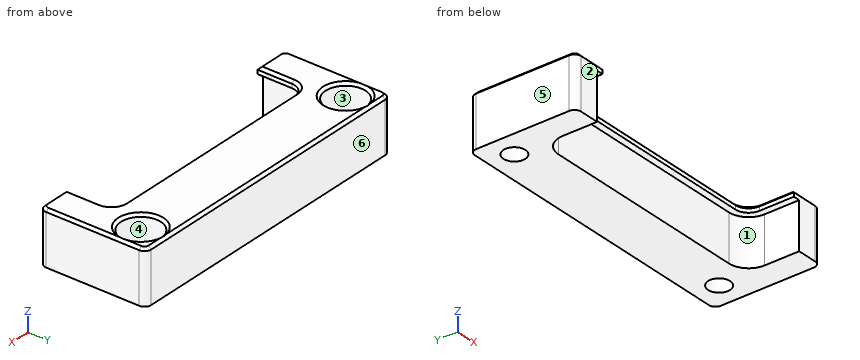
from build123d import *

# Parameters (mm, degrees)
BOSS_EXTRUDE1_DEPTH = 8
CUT_EXTRUDE1_REACH  = 51.356
SKETCH2_R           = 1.65
SKETCH3_R           = 3
CUT_EXTRUDE2_DEPTH  = 4.5
CUT_EXTRUDE3_DEPTH  = 7
FILLET1_R           = 1
CHAMFER2_SIZE       = 0.4


with BuildPart() as part:
    # Sketch1 → Boss-Extrude1 (new body)
    with BuildSketch(Plane.XY):
        with BuildLine():
            Line((0, 0), (0, 16))
            Line((0, 16), (46, 16))
            Line((46, 16), (46, 0))
            Line((46, 0), (41, 0))
            Line((41, 0), (41, 5.2))
            ThreePointArc((41, 5.2), (40.414213562, 6.614213562), (39, 7.2))
            Line((39, 7.2), (7, 7.2))
            ThreePointArc((7, 7.2), (5.585786438, 6.614213562), (5, 5.2))
            Line((5, 5.2), (5, 0))
            Line((5, 0), (0, 0))
        make_face()
    extrude(amount=BOSS_EXTRUDE1_DEPTH)

    # Sketch2 → Cut-Extrude1 (cut, up to next)
    with BuildSketch(Plane.XY.offset(8), mode=Mode.PRIVATE) as cut_extrude1_sk1:
        with Locations((3.75, 12.25)):
            Circle(SKETCH2_R)
    cut_extrude1_tool1 = extrude(cut_extrude1_sk1.sketch, amount=-CUT_EXTRUDE1_REACH, mode=Mode.PRIVATE) & part.part
    # Sketch2 → Cut-Extrude1 (cut, up to next)
    with BuildSketch(Plane.XY.offset(8), mode=Mode.PRIVATE) as cut_extrude1_sk2:
        with Locations((42.25, 12.25)):
            Circle(SKETCH2_R)
    cut_extrude1_tool2 = extrude(cut_extrude1_sk2.sketch, amount=-CUT_EXTRUDE1_REACH, mode=Mode.PRIVATE) & part.part
    add(cut_extrude1_tool1.solids().sort_by_distance((3.75, 12.25, 8))[0], mode=Mode.SUBTRACT)
    add(cut_extrude1_tool2.solids().sort_by_distance((42.25, 12.25, 8))[0], mode=Mode.SUBTRACT)

    # Sketch3 → Cut-Extrude2 (cut)
    with BuildSketch(Plane.XY.offset(8)):
        with Locations((3.75, 12.25)):
            Circle(SKETCH3_R)
        with Locations((42.25, 12.25)):
            Circle(SKETCH3_R)
    extrude(amount=-CUT_EXTRUDE2_DEPTH, mode=Mode.SUBTRACT)

    # Sketch4 → Cut-Extrude3 (cut)
    with BuildSketch(Plane(origin=(0, 0, 0), x_dir=(-1, 0, 0), z_dir=(0, 0, -1))):
        with BuildLine():
            Line((-4, 0), (-5, 0))
            Line((-5, 0), (-5, 5.2))
            ThreePointArc((-5, 5.2), (-5.585786438, 6.614213562), (-7, 7.2))
            Line((-7, 7.2), (-39, 7.2))
            ThreePointArc((-39, 7.2), (-40.414213592, 6.614213592), (-41, 5.2))
            Line((-41, 5.2), (-41, 0))
            Line((-41, 0), (-42, 0))
            Line((-42, 0), (-42, 5.200000101))
            ThreePointArc((-42, 5.200000101), (-41.121320373, 7.321320373), (-39.000000101, 8.2))
            Line((-39.000000101, 8.2), (-7, 8.2))
            ThreePointArc((-7, 8.2), (-4.878679656, 7.321320344), (-4, 5.2))
            Line((-4, 5.2), (-4, 0))
        make_face()
    extrude(amount=-CUT_EXTRUDE3_DEPTH, mode=Mode.SUBTRACT)

    # Fillet1
    fillet1_edges = [part.edges().sort_by_distance(p)[0] for p in [
        (0, 0, 4),
        (0, 16, 4),
        (46, 16, 4),
        (46, 0, 4),
    ]]
    fillet(fillet1_edges, radius=FILLET1_R)

    # Chamfer2
    # the kernel refuses this chamfer: 0.4 mm, written as the material it takes off along each edge
    with BuildSketch(Plane(origin=(6.028673195, 0, 8), x_dir=(0, 0.9996219169112966, 0.027495876610587326), z_dir=(-1, 0, 0)), Plane(origin=(45, 0, 8), x_dir=(0, 0.9996219169112966, 0.027495876610587378), z_dir=(-1, 0, 0))) as chamfer2_piece_1:
        Polygon((CHAMFER2_SIZE * 0.999621916911, CHAMFER2_SIZE * 0.0274958766106), (-CHAMFER2_SIZE * 0.0274958766106, CHAMFER2_SIZE * 0.999621916911), (0, 0), align=None)
    extrude(amount=5.028673195, mode=Mode.SUBTRACT)
    with BuildSketch(Plane(origin=(46, 15, 8), x_dir=(-0.9996219169112966, 0, 0.027495876610587656), z_dir=(0, -1, 0))) as chamfer2_piece_2:
        Polygon((CHAMFER2_SIZE * 0.999621916911, CHAMFER2_SIZE * 0.0274958766106), (-CHAMFER2_SIZE * 0.0274958766106, CHAMFER2_SIZE * 0.999621916911), (0, 0), align=None)
    extrude(amount=14, mode=Mode.SUBTRACT)
    with BuildSketch(Plane(origin=(1, 1, 8), x_dir=(-1, 0, 0), z_dir=(0, 1, 0))) as chamfer2_piece_3:
        Polygon((1, -CHAMFER2_SIZE), (1 - CHAMFER2_SIZE, 0), (1, 0), align=None)
    revolve(axis=Axis((1, 1, 8), (0, 0, 1)), revolution_arc=90, mode=Mode.SUBTRACT)
    with BuildSketch(Plane(origin=(45, 1, 8), x_dir=(1, 0, 0), z_dir=(0, 1, 0))) as chamfer2_piece_4:
        Polygon((1 - CHAMFER2_SIZE, 0), (1, CHAMFER2_SIZE), (1, 0), align=None)
    revolve(axis=Axis((45, 1, 8), (0, 0, -1)), revolution_arc=90, mode=Mode.SUBTRACT)
    with BuildSketch(Plane(origin=(45, 15, 8), x_dir=(0, 1, 0), z_dir=(-1, 0, 0))) as chamfer2_piece_5:
        Polygon((1 - CHAMFER2_SIZE, 0), (1, CHAMFER2_SIZE), (1, 0), align=None)
    revolve(axis=Axis((45, 15, 8), (0, 0, -1)), revolution_arc=90, mode=Mode.SUBTRACT)
    with BuildSketch(Plane(origin=(1, 15, 8), x_dir=(-1, 0, 0), z_dir=(0, -1, 0))) as chamfer2_piece_6:
        Polygon((1, CHAMFER2_SIZE), (1 - CHAMFER2_SIZE, 0), (1, 0), align=None)
    revolve(axis=Axis((1, 15, 8), (0, 0, -1)), revolution_arc=90, mode=Mode.SUBTRACT)
    with BuildSketch(Plane(origin=(7, 5.2, 8), x_dir=(0, 1, 0), z_dir=(1, 0, 0))) as chamfer2_piece_7:
        Polygon((2 + CHAMFER2_SIZE, 0), (2, -CHAMFER2_SIZE), (2, 0), align=None)
    revolve(axis=Axis((7, 5.2, 8), (0, 0, 1)), revolution_arc=90, mode=Mode.SUBTRACT)
    with BuildSketch(Plane(origin=(39, 7.2, 8), x_dir=(0, 0.9996219169112966, 0.027495876610587302), z_dir=(-1, 0, 0))) as chamfer2_piece_8:
        Polygon((CHAMFER2_SIZE * 0.999621916911, CHAMFER2_SIZE * 0.0274958766106), (-CHAMFER2_SIZE * 0.0274958766106, CHAMFER2_SIZE * 0.999621916911), (0, 0), align=None)
    extrude(amount=32, mode=Mode.SUBTRACT)
    with BuildSketch(Plane(origin=(39, 5.2, 8), x_dir=(1, 0, 0), z_dir=(0, -1, 0))) as chamfer2_piece_9:
        Polygon((2 + CHAMFER2_SIZE, 0), (2, -CHAMFER2_SIZE), (2, 0), align=None)
    revolve(axis=Axis((39, 5.2, 8), (0, 0, 1)), revolution_arc=90, mode=Mode.SUBTRACT)
    with BuildSketch(Plane(origin=(41, -1.028673195, 8), x_dir=(0.9996219169112966, 1.3659117145536696e-15, 0.027495876610587656), z_dir=(0, 1, 0)), Plane(origin=(5, 5.2, 8), x_dir=(-0.9996219169112966, 0, 0.027495876610587243), z_dir=(0, -1, 0))) as chamfer2_piece_10:
        Polygon((CHAMFER2_SIZE * 0.999621916911, CHAMFER2_SIZE * 0.0274958766106), (-CHAMFER2_SIZE * 0.0274958766106, CHAMFER2_SIZE * 0.999621916911), (0, 0), align=None)
    extrude(amount=6.228673195, mode=Mode.SUBTRACT)
    with BuildSketch(Plane(origin=(3.75, 12.25, 8), x_dir=(1, 0, 0), z_dir=(0, -1, 0))) as chamfer2_piece_11:
        Polygon((3 + CHAMFER2_SIZE, 0), (3, -CHAMFER2_SIZE), (3, 0), align=None)
    revolve(axis=Axis((3.75, 12.25, 8), (0, 0, 1)), mode=Mode.SUBTRACT)
    with BuildSketch(Plane(origin=(42.25, 12.25, 8), x_dir=(1, 0, 0), z_dir=(0, -1, 0))) as chamfer2_piece_12:
        Polygon((3 + CHAMFER2_SIZE, 0), (3, -CHAMFER2_SIZE), (3, 0), align=None)
    revolve(axis=Axis((42.25, 12.25, 8), (0, 0, 1)), mode=Mode.SUBTRACT)
    with BuildSketch(Plane(origin=(0, 1, 8), x_dir=(-0.027495876610586258, 0, -0.9996219169112966), z_dir=(0, 1, 0))) as chamfer2_piece_13:
        Polygon((CHAMFER2_SIZE * 0.999621916911, -CHAMFER2_SIZE * 0.0274958766106), (-CHAMFER2_SIZE * 0.0274958766106, -CHAMFER2_SIZE * 0.999621916911), (0, 0), align=None)
    extrude(amount=14, mode=Mode.SUBTRACT)
    with BuildSketch(Plane(origin=(1, 16, 8), x_dir=(0, -0.9996219169112966, 0.027495876610587302), z_dir=(1, 0, 0))) as chamfer2_piece_14:
        Polygon((CHAMFER2_SIZE * 0.999621916911, CHAMFER2_SIZE * 0.0274958766106), (-CHAMFER2_SIZE * 0.0274958766106, CHAMFER2_SIZE * 0.999621916911), (0, 0), align=None)
    extrude(amount=44, mode=Mode.SUBTRACT)


solid = part.part
Part model, mm, in its own coordinate system. Face numbers are marked on the shaded views. A direction names the side the tool comes from. Coordinates: 2 decimals unless noted, no trailing zeros. Write each loop counter-clockwise with the first axis right and the second up, starting at its lowest first coordinate (ties: lowest second). Pieces come first, ordered by that corner, then holes. Notation, with made-up numbers: M 46.25,37 L 95.25,37 A13 cw 95.25,61 Z; hole C -7,79 d2. An arc over 180 degrees is marked long. Return JSON: item names as keys, results as strings.
1. Probe L1, parallel to X at y = 14.75, z = 7; L2, parallel to X at y = 4.25, z = 3.5; L3, parallel to X at y = 2.25, z = 7.5. List the from-to ranges inside material, lowest first.
Determined:
{"L1": "0 to 2.09, 5.41 to 40.59, 43.91 to 46", "L2": "0 to 4, 42 to 46", "L3": "0 to 5, 41 to 46"}
2. Flat gauge pins, fed straight in: pin 1 Ø5.5 at (x, y) = (3.75, 12.25) entering from +Z; pin 2 Ø0.5 at (x, z) = (24, 7.5) entering from -Y; pin 3 Ø3 at (x, y) = (2.5, 11) entering from +Z. Where does each tip first touch, or does it go through?
Determined:
{"pin 1": "z = 3.5", "pin 2": "y = 7.2", "pin 3": "z = 7.87"}
3. Saw through at C-C, the plane x = 26.5. Write the cut outline in (y, z).
Determined:
{"outline": "M 7.2,7 L 8.2,7 L 8.2,0 L 16,0 L 16,7.6 L 15.6,8 L 7.6,8 L 7.2,7.6 Z"}
4. 3-axis set-ups, long thin cutter, end or side, ignore diameter. For the marked faces 1, 2 and 3: which of +Z, -Z, +X, -X, +Y, -Y reach the whole face in a straight line?
Determined:
{"face 1": "-Z, -Y", "face 2": "+Z, -Z, +X, -X, -Y", "face 3": "+Z"}
5. Saw through at A-A, the plane y = 2.5. Write the cut outline in (x, z).
Determined:
{"outline": "M 0,0 L 4,0 L 4,7 L 5,7 L 5,7.6 L 4.6,8 L 0.4,8 L 0,7.6 Z; M 41,7 L 42,7 L 42,0 L 46,0 L 46,7.6 L 45.6,8 L 41.4,8 L 41,7.6 Z"}
6. Saw through at B-B, the plane z = 0.75. Write the cut outline in (x, y), then the cut area to 3 significant figures.
Determined:
{"outline": "M 0,1 A1 ccw 1,0 L 4,0 L 4,5.2 A3 cw 7,8.2 L 39,8.2 A3 cw 42,5.2 L 42,0 L 45,0 A1 ccw 46,1 L 46,15 A1 ccw 45,16 L 1,16 A1 ccw 0,15 Z; hole C 3.75,12.25 d3.3; hole C 42.25,12.25 d3.3", "area": "410 mm²"}
7. Saw through at D-D, the plane y = 12.25. Write the cut outline in (x, z) (3 decimals), then the cut area to 3 significant figures.
Determined:
{"outline": "M 0,0 L 2.1,0 L 2.1,3.5 L 0.75,3.5 L 0.75,7.6 L 0.375,7.975 L 0,7.6 Z; M 5.4,0 L 40.6,0 L 40.6,3.5 L 39.25,3.5 L 39.25,7.6 L 38.85,8 L 7.15,8 L 6.75,7.6 L 6.75,3.5 L 5.4,3.5 Z; M 43.9,0 L 46,0 L 46,7.6 L 45.625,7.975 L 45.25,7.6 L 45.25,3.5 L 43.9,3.5 Z", "area": "290 mm²"}
8. Pull direction Y, two halves, no side cores. Call the marked faces 4, 5 and 6: pulls with the +Y half, pulls with the -Y half, needs draft (parallel to the pull), parting line crosses it, or undercut.
Determined:
{"face 4": "undercut", "face 5": "needs draft", "face 6": "pulls with the +Y half"}
